```python
from build123d import *

# Parameters (mm, degrees)
BOSS_EXTRUDE1_DEPTH = 711.2
FILLET1_R           = 10


with BuildPart() as part:
    # Sketch1 → Boss-Extrude1 (new body)
    with BuildSketch(Plane(origin=(0, 0, 0), x_dir=(0, 0, -1), z_dir=(1, 0, 0))):
        with BuildLine():
            Line((122.672579939, -32.870018728), (122.672579939, -22.870018728))
            ThreePointArc((122.672579939, -22.870018728), (59.787928159, -12.213574307), (0, 10))
            Line((0, 10), (0, 0))
            ThreePointArc((0, 0), (60.329037039, -20.194128476), (122.672579939, -32.870018728))
        make_face()
    extrude(amount=BOSS_EXTRUDE1_DEPTH)

    # Fillet1
    fillet1_edges = [part.edges().sort_by_distance(p)[0] for p in [
        (355.6, -22.870018728, -122.672579939),
    ]]
    fillet(fillet1_edges, radius=FILLET1_R)


solid = part.part
```
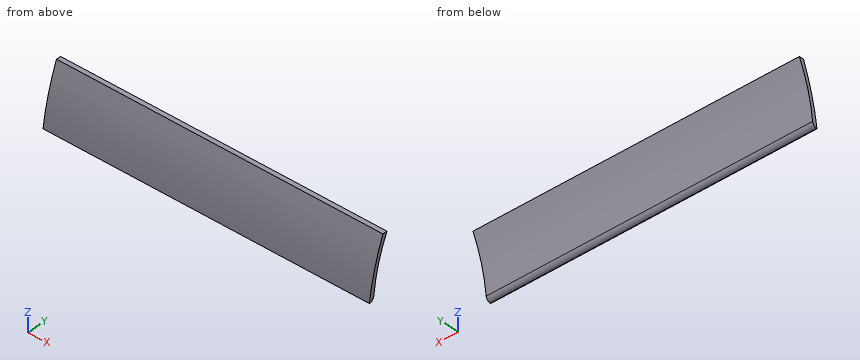
Source: CAD feature listing. Evaluate the final solid. Frame: model axes, mm. Round coordinates to 2 decimals unless told otherwise and drop trailing zeros. Order: outer loops, then holes, each group sorted by start corner. A loop starts at its lowest first (then second) coordinate and runs counter-clockwise, first axis right, second up. Notation, with made-up numbers: (1.25, 46.25) -> (36.25, 46.25) arc R29 cw to (36.25, 67.25) -> close; hole circle Ø3 at (60, 87). An arc over 180 degrees is marked (long way). Use CSV: the item, a comma, the result in double quotes.
(1) Section C-C on y = -14. Return the cut outline in (x, z).
Report:
outline,"(0, -66.75) -> (711.2, -66.75) -> (711.2, -39.04) -> (0, -39.04) -> close"
(2) Section B-B on z = -107. Return the cut outline in (x, y).
Report:
outline,"(0, -30.43) -> (711.2, -30.43) -> (711.2, -21.34) -> (0, -21.34) -> close"
(3) Section A-A on x = 550. Return the cut outline in (y, z).
Report:
outline,"(-32.87, -122.67) -> (-32.03, -122.67) arc R10 ccw to (-22.08, -113.68) arc R340 cw to (10, 0) -> (0, 0) arc R520 ccw to start"
(4) Ray query, L1, parallel to Z at x = 209.5, y = 4.5; L2, parallel to Y at x = 392, z = -81.5; L3, parallel to Y at x = 399.5, z = -115.5. Return the intervals inside material, ascending.
Report:
L1,"-11.98 to 0"
L2,"-25.39 to -17.27"
L3,"-31.81 to -22.44"
(5) First-contact query: pin 1 Ø1 at (x, z) = (428, -52) entering from -Y; pin 2 Ø1.5 at (x, y) = (267, 4) entering from -Z; pin 3 Ø1.5 at (x, y) = (377, 5.5) entering from -Z. Flat tips, straight axial feed; report the tip coordinate or a pass-through.
Report:
pin 1,"y = -18.03"
pin 2,"z = -14.89"
pin 3,"z = -11.41"
